from build123d import *

# Parameters (mm, degrees)
IZIM1_R                     = 2
IZIM1_W                     = 70
IZIM1_H                     = 18
Y_KSEKLIK_EKSTR_ZYON1_DEPTH = 3


with BuildPart() as part:
    # Çizim1 → Yükseklik-Ekstrüzyon1 (new body)
    # profile 1 of 2: a face of its own
    with BuildSketch(Plane.XY):
        Polygon((45, 63), (70, 18), (0, 18), (25, 63), align=None)
        with Locations((35, 53)):
            Circle(IZIM1_R, mode=Mode.SUBTRACT)
    # profile 2 of 2: a face of its own
    with BuildSketch(Plane.XY):
        with Locations((35, 9)):
            Rectangle(IZIM1_W, IZIM1_H)
        with Locations((35, 8)):
            Circle(IZIM1_R, mode=Mode.SUBTRACT)
    extrude(amount=Y_KSEKLIK_EKSTR_ZYON1_DEPTH)


solid = part.part
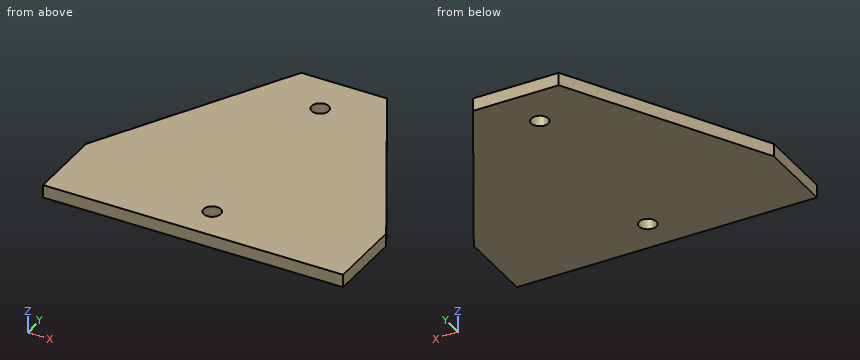
CAD build for the part. Positions are in the model's coordinates, mm. Give positions to 0.01 mm unless a question says otherwise; leave off trailing zeros. Loops run counter-clockwise (first coordinate to the right, second up) from the corner with the lowest first, then second, coordinate; pieces in that order, holes last. Notation, with made-up numbers: M -34,69.25 L -3,69.25 A19 ccw -3,94.25 Z; hole C 22,37.25 d4. An arc over 180 degrees is marked long. One line per question, with ' | ' between items. Start each with the question number.
1. Saw through at D-D on x = 58. Give the cut face in (y, z), plus the area to 3 significant figures.
2. Saw through at A-A on x = 35. Give the cut face in (y, z), plus the area to 3 significant figures.
3. Probe L1, parallel to Y at x = 35, z = 0.95; L2, parallel to Y at x = 33.5, z = 0.45; L3, parallel to X at y = 9.5, z = 1.85. List the from-to ranges inside material, lowest first. Write a range as from..to.
4. Saw through at C-C on y = 8. Give the cut face in (x, z).
5. Saw through at B-B on z = 0.7. Give the cut face in (x, y).
Result sheet:
1) outline: M 0,0 L 39.6,0 L 39.6,3 L 0,3 Z | area: 119 mm^2
2) outline: M 0,0 L 6,0 L 6,3 L 0,3 Z; M 10,0 L 51,0 L 51,3 L 10,3 Z; M 55,0 L 63,0 L 63,3 L 55,3 Z | area: 165 mm^2
3) L1: y = 0..6, 10..51, 55..63 | L2: y = 0..6.68, 9.32..51.68, 54.32..63 | L3: x = 0..33.68, 36.32..70
4) outline: M 0,0 L 33,0 L 33,3 L 0,3 Z; M 37,0 L 70,0 L 70,3 L 37,3 Z
5) outline: M 0,0 L 70,0 L 70,18 L 45,63 L 25,63 L 0,18 Z; hole C 35,8 d4; hole C 35,53 d4
